Here's the drawing with two shaded views (mm, measured from the low corner). I have some questions. Give positions to 0.01 mm unless a question says otherwise; leave off trailing zeros. Write each loop counter-clockwise with the first axis right and the second up, starting at its lowest first coordinate (ties: lowest second). Pieces come first, ordered by that corner, then holes. Notation, with made-up numbers: (11, 85) - (69, 85) arc R15 cw to (69, 91) - close; hole circle Ø7 at (45, 71). An arc over 180 degrees is marked (long way). Use one line per item in the form item = value.
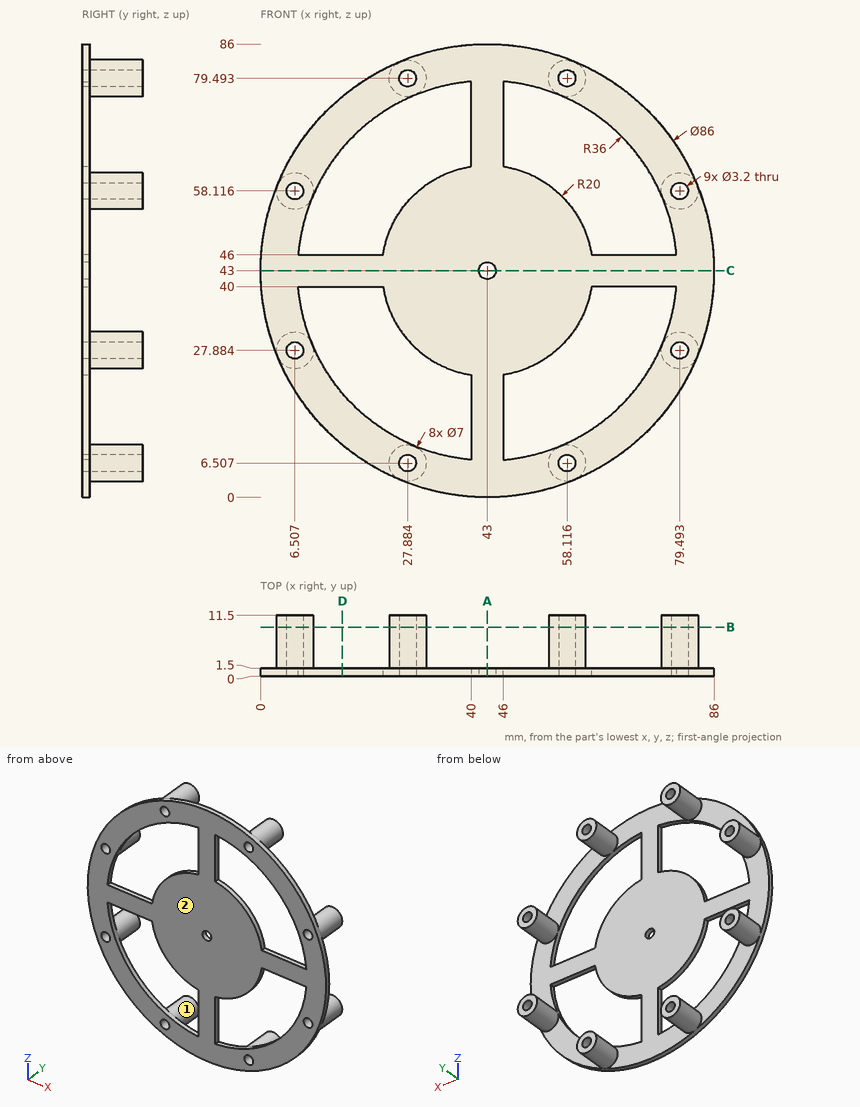
1. Imagine slicing it at C-C, the plane z = 43. List the corners of the cut face in (x, y) for me.
Response values:
outline = (0, 0) - (41.4, 0) - (41.4, 1.5) - (0, 1.5) - close; (44.6, 0) - (86, 0) - (86, 1.5) - (44.6, 1.5) - close
2. Imagine slicing it at B-B, the plane y = 9.25. State how many separate pieces and enclosed holes the cut face has.
Response values:
separate_pieces = 8
enclosed_holes = 8
3. If I drill on line 1 (X direction, y = 6.5, z = 31) (1 decimal); line 2 (X direction, y = 1.25, z = 43), over which ranges is the centre line in solid material (lowest first)? Write a range as from..to.
Response values:
line_1 = 4.9..8.1, 77.9..81.1
line_2 = 0..41.4, 44.6..86
4. If we mould it in two halves opening along X, with no side actions, what happens to the marked faces 1 and 2? For each: pulls with the +X half, pulls with the -X half, needs draft (parallel to the pull), parting line crosses it, or undercut.
Response values:
face_1 = undercut
face_2 = needs draft
5. Imagine slicing it at D-D, the plane x = 15.5. List the corners of the cut face in (y, z) for me.
Response values:
outline = (0, 9.94) - (1.5, 9.94) - (1.5, 19.77) - (0, 19.77) - close; (0, 40) - (1.5, 40) - (1.5, 46) - (0, 46) - close; (0, 66.23) - (1.5, 66.23) - (1.5, 76.06) - (0, 76.06) - close
6. For pin 1 (2 mm diameter, centred on x = 76, y = 4, fed in from +Z); pin 2 (1 mm diameter, centred on x = 42, z = 64.5, fed in from +Y); pin 3 (0.8 mm diameter, centred on x = 69, y = 1, fed in from -Z); pin 4 (5 mm diameter, centred on x = 58.12, z = 6.51, fed in from -Y), each with a flat end and sliding along its axis, tell me the tip position at first contact or that it passes through.
Response values:
pin_1 = 60.57
pin_2 = 1.5
pin_3 = 8.45
pin_4 = 0
7. Imagine slicing it at A-A, the plane x = 43. List the corners of the cut face in (y, z) for me, and give its area (3 significant figures).
Response values:
outline = (0, 0) - (1.5, 0) - (1.5, 41.4) - (0, 41.4) - close; (0, 44.6) - (1.5, 44.6) - (1.5, 86) - (0, 86) - close
area = 124 mm²
